Autodesk Inventor part; units mm, degrees
ref_plane "YZ Plane" through (0, 0, 0) normal (1, 0, 0) x (0, 1, 0)
ref_plane "XZ Plane" through (0, 0, 0) normal (0, 1, 0) x (-1, 0, 0)
ref_plane "XY Plane" through (0, 0, 0) normal (0, 0, 1) x (1, 0, 0)
sketch "Sketch1" plane through (0, 0, 0) normal (1, 0, 0) x (0, 1, 0)
  line L0 (19.8793, 20.7795) -> (-17.4785, 20.7795)
  line L1 (-17.4785, 20.7795) -> (-17.4785, -16.5784)
  line L2 (-17.4785, -16.5784) -> (19.8793, -16.5784)
  line L3 (19.8793, -16.5784) -> (19.8793, 20.7795)
  circle A0 centre (19.8793, 20.7795) radius 4.8895
  circle A1 centre (19.8793, -16.5784) radius 4.8895
  circle A2 centre (-17.4785, -16.5784) radius 4.8895
  circle A3 centre (-17.4785, 20.7795) radius 4.8895
  line L4 (32.5793, 39.8295) -> (-30.1785, 39.8295)
  line L5 (-30.1785, 39.8295) -> (-30.1785, -45.1534)
  line L6 (-30.1785, -45.1534) -> (32.5793, -45.1534)
  line L7 (32.5793, -45.1534) -> (32.5793, 39.8295)
  circle A4 centre (19.8793, 20.7795) radius 2.4575
  circle A5 centre (19.8793, -16.5784) radius 2.4575
  circle A6 centre (-17.4785, -16.5784) radius 2.4575
  circle A7 centre (-17.4785, 20.7795) radius 2.4575
  point P0 (0, 0)
  dimension "d0" = 9.779
  dimension "d4" = 52.832
  dimension "d5" = 12.7
  dimension "d6" = 19.05
  dimension "d7" = 12.7
  dimension "d8" = 28.575
  dimension "d13" = 4.9149
extrude "Extrusion1" add sketch "Sketch1" along normal blind 6.35 contours A3 L1 A7 L0 | L0 A7 L1 A3 | L0 A0 L3 A1 L2 A2 L1 A3 | A7 L1 L0 | L0 L1 A7 | A0 L3 A4 L0 | L0 A4 L3 A0 | A4 L3 L0 | L0 L3 A4 | A2 L2 A6 L1 | L1 A6 L2 A2 | A1 L2 A5 L3 | L3 A5 L2 A1 | A6 L2 L1 | L1 L2 A6 | A5 L2 L3 | L3 L2 A5 | L7 L6 L5 L4
extrude "Extrusion2" add sketch "Sketch1" along normal blind 12.7 contours A3 L1 A7 L0 | L0 A7 L1 A3 | A7 L1 L0 | L0 L1 A7 | A1 L2 A5 L3 | L3 A5 L2 A1 | A5 L2 L3 | L3 L2 A5
extrude "Extrusion3" cut sketch "Sketch1" along normal blind 12.7 contours A7 L1 L0 | L0 L1 A7 | A5 L2 L3 | L3 L2 A5
sketch "Sketch2" plane through (0, -30.1785, -45.1534) normal (0, 0, -1) x (-1, 0, 0)
  line L0 (0, 0) -> (-6.35, 0)
  line L1 (0, 0) -> (-50.8, 0)
  line L2 (-50.8, 0) -> (-50.8, 62.7579)
  line L3 (-50.8, 62.7579) -> (0, 62.7579)
  line L4 (0, 62.7579) -> (0, 0)
  line L5 (0, 62.7579) -> (-6.35, 62.7579)
  line L6 (-50.8, 62.7579) -> (-25.4, 77.4226)
  line L7 (-25.4, 77.4226) -> (0, 62.7579)
  line L8 (-50.8, 62.7579) -> (0, 62.7579)
  point P0 (0, 30.1785)
  dimension "d16" = 50.8
  dimension "d89" = 30
  dimension "d90" = 30
extrude "Extrusion4" add sketch "Sketch2" along normal blind 6.35
sketch "Sketch4" plane through (0, 32.5793, 39.8295) normal (0, 1, 0) x (1, 0, 0)
  line L0 (0, 84.9829) -> (0, 0)
  line L1 (0, 0) -> (6.35, 0)
  line L2 (6.35, 84.9829) -> (6.35, 0)
  line L3 (0, 78.6329) -> (6.35, 78.6329)
  line L4 (6.35, 78.6329) -> (6.35, 129.4329)
  line L5 (6.35, 129.4329) -> (0, 129.4329)
  line L6 (0, 129.4329) -> (0, 78.6329)
  line L7 (6.35, 129.4329) -> (50.8, 129.4329)
  line L8 (50.8, 129.4329) -> (50.8, 123.0829)
  line L9 (50.8, 123.0829) -> (6.35, 123.0829)
  line L10 (6.35, 123.0829) -> (6.35, 129.4329)
  line L11 (0, 84.9829) -> (6.35, 84.9829)
  point P0 (0, 39.8295)
  dimension "d25" = 6.35
  dimension "d26" = 50.8
  dimension "d27" = 6.35
sketch "Sketch3" plane through (0, -30.1785, -45.1534) normal (0, 0, 1) x (1, 0, 0)
  circle A0 centre (24.1046, 36.4435) radius 9.7536
  line L0 (6.35, 62.7579) -> (6.35, 0)
  circle A1 centre (24.1046, 36.4435) radius 14.2494
  line L1 (6.35, 0) -> (50.8, 0)
  point P0 (0, 30.1785)
  dimension "d19" = 19.5072
  dimension "d20" = 17.7546
  dimension "d22" = 28.4988
  dimension "d91" = 36.4435
extrude "Extrusion5" cut sketch "Sketch3" against normal blind 63.5 contours A0 | A1
sketch "Sketch5" plane through (0, -30.1785, -45.1534) normal (0, 0, 1) x (1, 0, 0)
  circle A0 centre (24.1046, 36.4435) radius 14.2494
  circle A1 centre (23.8385, 68.1924) radius 2.4574
  circle A2 centre (43.1546, 11.0435) radius 2.4574
  circle A3 centre (11.6326, 7.2457) radius 2.4574
  point P0 (0, 30.1785)
  dimension "d33" = 4.9149
  dimension "d46" = 31.75
  dimension "d47" = 31.75
  dimension "d48" = 31.75
  dimension "d49" = 31.75
  dimension "d50" = 60.325
  dimension "d51" = 25.4
extrude "Extrusion7" cut sketch "Sketch5" against normal blind 25.4 contours A1 | A2 | A3
ref_plane "Work Plane1" through (-9.525, -30.1785, 2.2051) normal (-1, 0, 0) x (0, 0, 1)
sketch "Sketch10" plane through (0, 0, 0) normal (-1, 0, 0) x (0, 0, 1)
  line L0 (14.9051, -30.1785) -> (14.9051, 32.5793)
  line L1 (14.9051, 32.5793) -> (2.2051, 32.5793)
  circle A0 centre (8.5551, 26.2293) radius 2.4574
  circle A1 centre (8.5551, 13.5293) radius 2.4574
  circle A2 centre (8.5551, 0.8293) radius 2.4574
  circle A3 centre (8.5551, -11.8707) radius 2.4574
  circle A4 centre (8.5551, -24.5707) radius 2.4574
  point P0 (0, 0)
  dimension "d77" = 4.9149
  dimension "d78" = 6.35
  dimension "d79" = 6.35
  dimension "d82" = 12.7
extrude "Extrusion12" cut sketch "Sketch10" against normal blind 25.4
sketch "Sketch11" plane through (0, -30.1785, -45.1534) normal (0, 0, 1) x (1, 0, 0)
  line L0 (52.0296, 47.0435) -> (52.0296, 15.1435)
  line L1 (46.7796, 15.1435) -> (46.7796, 47.0435)
  line L2 (52.0296, 15.1435) -> (46.7796, 15.1435)
  line L3 (46.7796, 47.0435) -> (52.0296, 47.0435)
  line L4 (46.2716, 47.5515) -> (46.2716, 14.6355)
  line L5 (46.2716, 14.6355) -> (52.5376, 14.6355)
  line L6 (52.5376, 14.6355) -> (52.5376, 47.5515)
  line L7 (52.5376, 47.5515) -> (46.2716, 47.5515)
  point P0 (0, 30.1785)
  dimension "d92" = 0.508
extrude "Extrusion13" cut sketch "Sketch11" against normal blind 25.4 contours L0 L2 L1 L3 | L7 L6 L5 L4
sketch "Sketch12" plane through (6.35, 0, 0) normal (1, 0, 0) x (0, 0, -1)
  line L0 (51.5034, 20.5143) -> (51.5034, -7.9845)
  line L1 (45.1534, -7.9845) -> (45.1534, 20.5143)
  line L2 (45.1534, 6.2649) -> (-81.3629, 6.2649)
  circle A0 centre (-33.4795, 18.9649) radius 2.3495
  circle A1 centre (-33.4795, -6.4351) radius 2.3495
  line L3 (-39.8295, 32.5793) -> (-39.8295, -30.1785)
  point P0 (0, 0)
  dimension "d95" = 4.699
  dimension "d96" = 4.699
  dimension "d97" = 12.7
  dimension "d98" = 12.7
  dimension "d99" = 6.35
extrude "Extrusion14" cut sketch "Sketch12" against normal blind 25.4
equation "\"d90\" = d89"
equation "\"d27\" = d25"
equation "\"d1\" = d0"
properties part number "motor mount 2" material "ABS Plastic"
Input: part model. Units: mm. Frame: model coordinates. A direction names the side the tool comes from. Coordinates: 2 decimals unless noted, no trailing zeros. Order: outer loops, then holes, each group sorted by start corner. A loop starts at its lowest first (then second) coordinate and runs counter-clockwise, first axis right, second up. Notation, with made-up numbers: M 29,66.5 L 55,66.5 A14 ccw 55,74.5 Z; hole C 29.25,25 d9. An arc over 180 degrees is marked long. Answer in a Markdown table with one row per item.
(1) Section query C-C, the plane z = -13. Output: boundary loops of the cut face in (x, y), plus the area to 3 significant figures.
Numbers:
| item | result |
|---|---|
| outline | M 0,-30.18 L 6.35,-30.18 L 6.35,16.55 L 12.7,16.55 L 12.7,23.21 L 6.35,23.21 L 6.35,32.58 L 0,32.58 Z |
| area | 441 mm^2 |
(2) Access query for faces 1 (the flat face through (12.7, -20, 20)), 2 (the flat face through (46.272, 1, -48)), 3 (the cylindrical face through (3.13, 24.05, 9.69)), 4 (the cylindrical face through (12.77, -25.11, -48.28)), 5 (the cylindrical face through (41.204, -20.63, -48.284)). Directions: +Z, -Z, +X, -X, +Y, -Y. A direction counts if a zero-diameter tool reaches every point of the face in a straight line with its end or side. Return the directions, or none.
Numbers:
| item | result |
|---|---|
| face 1 | +Z, +X, +Y, -Y |
| face 2 | +Z, -Z, +X |
| face 3 | +X, -X |
| face 4 | -Z |
| face 5 | +Z, -Z |
(3) Draft query along Z for faces 6 (the flat face through (6.35, 1, -2)), 7 (the cylindrical face through (21.888, 36.519, -48.284)), 8 (the flat face through (25.8, -8.1, -51.503)), 9 (the cylindrical face through (6.261, -16.345, 22.96)). Return one class per face: pulls with the +Z half, pulls with the -Z half, needs draft (parallel to the pull), parting line crosses it, or undercut.
Numbers:
| item | result |
|---|---|
| face 6 | undercut |
| face 7 | needs draft |
| face 8 | pulls with the -Z half |
| face 9 | undercut |
(4) Section query D-D, the plane x = 43. Output: boundary loops of the cut face in (y, z), plus the area to 3 significant figures.
Numbers:
| item | result |
|---|---|
| outline | M -30.18,-51.5 L -21.59,-51.5 L -21.59,-45.15 L -30.18,-45.15 Z; M -16.68,-51.5 L 37.08,-51.5 L 37.08,-45.15 L -16.68,-45.15 Z |
| area | 396 mm^2 |
(5) Contact query for flat-ended pins moving along their axis: pin 1 Ø4.5 at (y, z) = (13.53, 8.56) entering from +X; pin 2 Ø3 at (y, z) = (-5, 7.5) entering from +X; pin 3 Ø8 at (y, z) = (20.5, -14.5) entering from +X; pin 4 Ø1.4 at (x, z) = (48.5, -47) entering from +Y. Output: stop coordinate, or through.
Numbers:
| item | result |
|---|---|
| pin 1 | passes through |
| pin 2 | stops at x = 6.35 |
| pin 3 | stops at x = 12.7 |
| pin 4 | stops at y = 34.31 |
(6) Section query A-A, the plane x = 11.5. Output: boundary loops of the cut face in (y, z) (1 decimal), plus the area to 3 significant figures.
Numbers:
| item | result |
|---|---|
| outline | M -30.2,-51.5 L -25.4,-51.5 L -25.4,-45.2 L -30.2,-45.2 Z; C -17.5,20.8 d9.8; M -20.5,-51.5 L -0.4,-51.5 L -0.4,-45.2 L -20.5,-45.2 Z; M 12.9,-51.5 L 39.2,-51.5 L 39.2,-45.2 L 12.9,-45.2 Z; C 19.9,-16.6 d9.8; hole C -17.5,20.8 d4.9; hole C 19.9,-16.6 d4.9 |
| area | 437 mm^2 |
(7) Section query B-B, the plane x = 36.5. Output: boundary loops of the cut face in (y, z), plus the area to 3 significant figures.
Numbers:
| item | result |
|---|---|
| outline | M -30.18,-51.5 L -0.76,-51.5 L -0.76,-45.15 L -30.18,-45.15 Z; M 13.29,-51.5 L 40.84,-51.5 L 40.84,-45.15 L 13.29,-45.15 Z |
| area | 362 mm^2 |
(8) Material intervals for line 1 (Z direction, x = 7, y = 22); line 2 (X direction, y = -10.5, z = -44); line 3 (Z direction, x = 13.5, y = -17.5), sorted ascending. Write a range as [from, to].
Numbers:
| item | result |
|---|---|
| line 1 | z = [-51.5, -45.15], [-20.98, -17.82], [-15.34, -12.17] |
| line 2 | x = [0, 6.35] |
| line 3 | z = [-51.5, -45.15] |
